from build123d import *

# Parameters (mm, degrees)
SKETCH2_W           = 177.8
SKETCH2_H           = 101.6
BOSS_EXTRUDE3_DEPTH = 6.35
SKETCH3_R           = 9
SKETCH3_R_2         = 2.54
CUT_EXTRUDE1_DEPTH  = 103.587389576
SKETCH7_W           = 6.35
SKETCH7_H           = 14
SKETCH7_W_2         = 14
SKETCH7_H_2         = 6.35
CUT_EXTRUDE2_DEPTH  = 103.587389576
SKETCH9_W           = 5
SKETCH9_H           = 3
CUT_EXTRUDE3_DEPTH  = 103.587389576


with BuildPart() as part:
    # Sketch2 → Boss-Extrude3 (new body)
    with BuildSketch(Plane.XY):
        Rectangle(SKETCH2_W, SKETCH2_H)
    extrude(amount=BOSS_EXTRUDE3_DEPTH)

    # Sketch3 → Cut-Extrude1 (cut, through all)
    with BuildSketch(Plane.XY.offset(6.35)):
        with Locations((-9.4120506, 0)):
            Circle(SKETCH3_R)
        with Locations((-42.64375, 0)):
            Circle(SKETCH3_R)
        with Locations((-66.216922318, 23.573172318)):
            Circle(SKETCH3_R_2)
        with Locations((-19.070577682, 23.573172318)):
            Circle(SKETCH3_R_2)
        with Locations((-66.216922318, -23.573172318)):
            Circle(SKETCH3_R_2)
        with Locations((-19.070577682, -23.573172318)):
            Circle(SKETCH3_R_2)
        with Locations((45.9739194, 0)):
            Circle(SKETCH3_R)
    extrude(amount=-CUT_EXTRUDE1_DEPTH, mode=Mode.SUBTRACT)

    # Sketch7 → Cut-Extrude2 (cut, through all)
    with BuildSketch(Plane.XY.offset(6.35)):
        with Locations((-85.725, 0)):
            Rectangle(SKETCH7_W, SKETCH7_H)
        Polygon((-74.9, 50.8), (-88.9, 50.8), (-88.9, 37.554527849), (-82.55, 37.554527849), (-82.55, 44.45), (-74.9, 44.45), align=None)
        Polygon((-88.9, -38.1), (-88.9, -50.8), (-74.9, -50.8), (-74.9, -44.45), (-82.55, -44.45), (-82.55, -38.1), align=None)
        with Locations((63.509, 47.625)):
            Rectangle(SKETCH7_W_2, SKETCH7_H_2)
        with Locations((0, 47.625)):
            Rectangle(SKETCH7_W_2, SKETCH7_H_2)
        Polygon((88.9, 50.8), (83.9, 50.8), (83.9, 44.45), (75.9, 44.45), (75.9, -44.45), (83.9, -44.45), (83.9, -50.8), (88.9, -50.8), align=None)
        with Locations((63.509, -47.625)):
            Rectangle(SKETCH7_W_2, SKETCH7_H_2)
        with Locations((0, -47.625)):
            Rectangle(SKETCH7_W_2, SKETCH7_H_2)
    extrude(amount=-CUT_EXTRUDE2_DEPTH, mode=Mode.SUBTRACT)

    # Sketch9 → Cut-Extrude3 (cut, through all)
    with BuildSketch(Plane.XY.offset(6.35)):
        with Locations((61.062890697, 32.715)):
            Rectangle(SKETCH9_W, SKETCH9_H)
        with Locations((32.943445348, 32.715)):
            Rectangle(SKETCH9_W, SKETCH9_H)
        with Locations((61.063445348, -26.465)):
            Rectangle(SKETCH9_W, SKETCH9_H)
        with Locations((61.063445348, -32.715)):
            Rectangle(SKETCH9_W, SKETCH9_H)
        with Locations((32.943445348, -26.465)):
            Rectangle(SKETCH9_W, SKETCH9_H)
        with Locations((32.943445348, -32.715)):
            Rectangle(SKETCH9_W, SKETCH9_H)
        with Locations((70.509, -41.147)):
            Rectangle(SKETCH9_W, SKETCH9_H)
        with Locations((70.508445348, 41.147)):
            Rectangle(SKETCH9_W, SKETCH9_H)
        with Locations((70.508445348, 34.897)):
            Rectangle(SKETCH9_W, SKETCH9_H)
        with Locations((42.388445348, 41.147)):
            Rectangle(SKETCH9_W, SKETCH9_H)
        with Locations((42.388445348, 34.897)):
            Rectangle(SKETCH9_W, SKETCH9_H)
        with Locations((42.388445348, -34.897)):
            Rectangle(SKETCH9_W, SKETCH9_H)
        with Locations((42.388445348, -41.147)):
            Rectangle(SKETCH9_W, SKETCH9_H)
        with Locations((61.062890697, 26.465)):
            Rectangle(SKETCH9_W, SKETCH9_H)
        with Locations((32.943445348, 26.465)):
            Rectangle(SKETCH9_W, SKETCH9_H)
        with Locations((70.509, -34.897)):
            Rectangle(SKETCH9_W, SKETCH9_H)
    extrude(amount=-CUT_EXTRUDE3_DEPTH, mode=Mode.SUBTRACT)


solid = part.part
Source: CAD feature listing. Evaluate the final solid. Frame: model axes, mm. A direction names the side the tool comes from. Coordinates: 2 decimals unless noted, no trailing zeros. Order: outer loops, then holes, each group sorted by start corner. A loop starts at its lowest first (then second) coordinate and runs counter-clockwise, first axis right, second up.
Item 1: Cut plane C-C (z = 4.5). Count the separate pieces of the cut face and the enclosed holes in it, plus the area to 3 significant figures.
Output values:
separate pieces: 1
enclosed holes: 23
area: 15,100 mm2
Item 2: Pull-direction query (Y, two-part tool) for faces 5 (the face through (-79, 44.45, 3)), 6 (the face through (70, -39.647, 3)), 7 (the face through (70.509, 48, 3)); classes: pulls with the +Y half, pulls with the -Y half, needs draft (parallel to the pull), parting line crosses it, or undercut.
Output values:
face 5: pulls with the +Y half
face 6: undercut
face 7: needs draft
Item 3: First-contact query: P1, Ø1.5, axis at y = -34.5, z = 3.5, coming from the +X side; P2, Ø1.5, axis at x = -1.5, z = 4, coming from the -Y side. Flat tips, straight axial feed; report the tip coordinate or a pass-through.
Output values:
P1: stops at x = 75.9
P2: stops at y = -44.45
Item 4: Material intervals for line 1 (X direction, y = -42, z = 0.5); line 2 (X direction, y = 0.5, z = 5); line 3 (Y direction, x = -20, z = 4), sorted ascending.
Output values:
line 1: x = -82.55 to 39.89, 44.89 to 68.01, 73.01 to 75.9
line 2: x = -82.55 to -51.63, -33.66 to -18.4, -0.43 to 36.99, 54.96 to 75.9
line 3: y = -50.8 to -25.94, -21.21 to 21.21, 25.94 to 50.8
Item 5: Cut plane B-B (x = -4). Return loops of the section in (y, z), plus the area to 3 significant figures.
Output values:
outline: (-44.45, 0) - (-7.19, 0) - (-7.19, 6.35) - (-44.45, 6.35) - close; (7.19, 0) - (44.45, 0) - (44.45, 6.35) - (7.19, 6.35) - close
area: 473 mm2
Item 6: Cut plane A-A (y = 0). Return loops of the section in (x, z).
Output values:
outline: (-82.55, 0) - (-51.64, 0) - (-51.64, 6.35) - (-82.55, 6.35) - close; (-33.64, 0) - (-18.41, 0) - (-18.41, 6.35) - (-33.64, 6.35) - close; (-0.41, 0) - (36.97, 0) - (36.97, 6.35) - (-0.41, 6.35) - close; (54.97, 0) - (75.9, 0) - (75.9, 6.35) - (54.97, 6.35) - close
Item 7: Set-up query: faces 1 (the face through (7, 48, 3)), 2 (the face through (-82.55, 0, 3)), 3 (the face through (80, 44.45, 3)), 4 (the face through (70, 33.397, 3)). Return all of +Z, -Z, +X, -X, +Y, -Y with unobstructed straight access to the full face (end or side cutting, diameter ignored); none if empty.
Output values:
face 1: +Z, -Z, +Y
face 2: +Z, -Z, -X
face 3: +Z, -Z, +X
face 4: +Z, -Z
